```python
from build123d import *

# Parameters (mm, degrees)
SKETCH1_R           = 27.8
SKETCH1_R_2         = 8.3
SKETCH1_R_3         = 10.5
BOSS_EXTRUDE1_DEPTH = 16


with BuildPart() as part:
    # Sketch1 → Boss-Extrude1 (new body)
    with BuildSketch(Plane(origin=(0, 0, 0), x_dir=(-1, 0, 0), z_dir=(0, 1, 0))):
        Polygon((-320, 75), (320, 75), (320, 0), (47.5, -500), (-47.5, -500), (-320, 0), align=None)
        with Locations(Location((0, 0, 0), (0, 0, 90))):
            Circle(SKETCH1_R, mode=Mode.SUBTRACT)
        with Locations(Location((0, -425, 0), (0, 0, 90))):
            Circle(SKETCH1_R, mode=Mode.SUBTRACT)
        with Locations(Location((-40, -50, 0), (0, 0, 90))):
            Circle(SKETCH1_R_2, mode=Mode.SUBTRACT)
        with Locations(Location((40, -50, 0), (0, 0, 270))):
            Circle(SKETCH1_R_2, mode=Mode.SUBTRACT)
        with Locations(Location((-40, -380, 0), (0, 0, 90))):
            Circle(SKETCH1_R_2, mode=Mode.SUBTRACT)
        with Locations(Location((40, -380, 0), (0, 0, 270))):
            Circle(SKETCH1_R_2, mode=Mode.SUBTRACT)
        with Locations(Location((-280, 37.5, 0), (0, 0, 90))):
            Circle(SKETCH1_R_3, mode=Mode.SUBTRACT)
        with Locations(Location((280, 37.5, 0), (0, 0, 270))):
            Circle(SKETCH1_R_3, mode=Mode.SUBTRACT)
        with Locations(Location((-125, -285, 0), (0, 0, 90))):
            Circle(SKETCH1_R_3, mode=Mode.SUBTRACT)
        with Locations(Location((125, -285, 0), (0, 0, 270))):
            Circle(SKETCH1_R_3, mode=Mode.SUBTRACT)
    extrude(amount=BOSS_EXTRUDE1_DEPTH)


solid = part.part
```
Geometry check sheet. Reference: the model listing, model coordinates, mm. Coordinates: 2 decimals unless noted, no trailing zeros. Loops run counter-clockwise (first coordinate to the right, second up) from the corner with the lowest first, then second, coordinate; pieces in that order, holes last.
Item 1: Sectioned sample at D-D, the plane z = -422. Record the boundary of the cut face in (x, y), then the cut area to 3 significant figures.
Item 2: Go/stop test with flat-tipped pins: pin 1 Ø5 at (y, z) = (14, -309) entering from -X; pin 2 Ø17 at (x, z) = (-280, 37.5) entering from +Y; pin 3 Ø3 at (y, z) = (7.5, -242.5) entering from +X (3 decimals); pin 4 Ø8 at (x, y) = (-223.5, 4) entering from -Z. Record where each tip stops, or that it passes through.
Item 3: Thickness scan on line 1 (X direction, y = 11.25, z = 37.5); line 2 (X direction, y = 3.75, z = -50); line 3 (Z direction, x = 10.5, y = 13.5). Record the ranges inside material, lowest first.
Item 4: Release check for a two-part mould opening along Z. For faces 1 (the face through (-4, 16, -145)), 2 (the face through (31.897, 7.888, -51.799)), 3 (the face through (181.843, 7.888, -253.5)) record: released by +Z, released by -Z, zero draft, split by the parting line, or undercut.
Item 5: Sectioned sample at B-B, the plane z = -50. Record the boundary of the cut face in (x, y), then the cut area to 3 significant figures.
Item 6: Sectioned sample at A-A, the plane x = 40. Record the boundary of the cut face in (y, z).
Item 7: Sectioned sample at C-C, the plane y = 4.5. Count the separate pieces of the cut face and the enclosed holes in it, then the cut area to 3 significant figures.
Check result:
1. outline: (-90.01, 0) - (-27.64, 0) - (-27.64, 16) - (-90.01, 16) - close; (27.64, 0) - (90.01, 0) - (90.01, 16) - (27.64, 16) - close
1. area: 2,000 mm2
2. pin 1: stops at x = -152.96
2. pin 2: passes through
2. pin 3: stops at x = 188.655
2. pin 4: stops at z = -184.4
3. line 1: x = -320 to -290.5, -269.5 to 269.5, 290.5 to 320
3. line 2: x = -292.75 to -48.3, -31.7 to 31.7, 48.3 to 292.75
3. line 3: z = -500 to -450.74, -399.26 to -25.74, 25.74 to 75
4. face 1: zero draft
4. face 2: undercut
4. face 3: released by -Z
5. outline: (-292.75, 0) - (-48.3, 0) - (-48.3, 16) - (-292.75, 16) - close; (-31.7, 0) - (31.7, 0) - (31.7, 16) - (-31.7, 16) - close; (48.3, 0) - (292.75, 0) - (292.75, 16) - (48.3, 16) - close
5. area: 8,840 mm2
6. outline: (0, -500) - (16, -500) - (16, -388.3) - (0, -388.3) - close; (0, -371.7) - (16, -371.7) - (16, -58.3) - (0, -58.3) - close; (0, -41.7) - (16, -41.7) - (16, 75) - (0, 75) - close
7. separate pieces: 1
7. enclosed holes: 10
7. area: 225,000 mm2
